Geometry: see drawing. Coordinates: mm, zero at the bounding-box minimum. Coordinates: 2 decimals unless noted, no trailing zeros. Write each loop counter-clockwise with the first axis right and the second up, starting at its lowest first coordinate (ties: lowest second). Pieces come first, ordered by that corner, then holes. Notation, with made-up numbers: (89.5, 62) - (148.5, 62) arc R18 cw to (148.5, 87) - close; hole circle Ø6 at (-19, 28). An arc over 180 degrees is marked (long way). One line per question, with ' | ' between items. Start each with the question number.
1) Section query C-C on y = 39.5. Return loops of the section in (x, z), and give its area (3 significant figures).
2) Section query B-B on z = 228. Return loops of the section in (x, y), and give its area (3 significant figures).
3) First-contact query: P1, Ø1, axis at x = 1, z = 157, coming from the +Y side. Flat tip, straight axial feed; report the tip coordinate or a pass-through.
4) Line query: line 1 (Y direction, x = 3.75, z = 120); line 2 (Y direction, x = 1.35, z = 216); line 3 (Z direction, x = 1.15, y = 46). Output: solid intervals per line, ascending.
5) Section query A-A on x = 4.05. Return loops of the section in (y, z) (1 decimal), and give its area (3 significant figures).
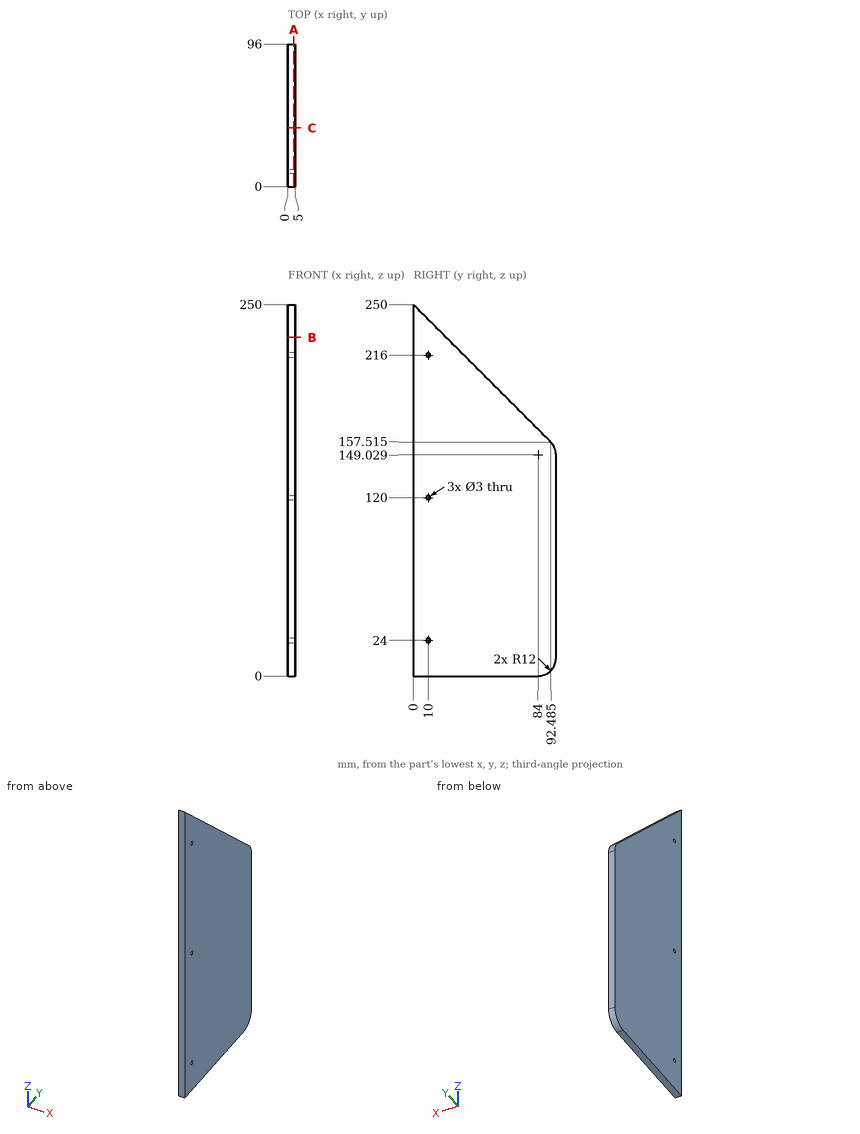
Answer key:
1) outline: (0, 0) - (5, 0) - (5, 210.5) - (0, 210.5) - close | area: 1,050 mm²
2) outline: (0, 0) - (5, 0) - (5, 22) - (0, 22) - close | area: 110 mm²
3) P1: y = 93.39
4) line 1: 0 to 8.5, 11.5 to 96 | line 2: 0 to 8.5, 11.5 to 34 | line 3: 0 to 204
5) outline: (0, 0) - (84, 0) arc R12 ccw to (96, 12) - (96, 149) arc R12 ccw to (92.5, 157.5) - (0, 250) - close; hole circle Ø3 at (10, 24); hole circle Ø3 at (10, 120); hole circle Ø3 at (10, 216) | area: 19,300 mm²
